Check sheet for the drawn part. Datum: minimum x, y, z corner. Units: mm. Give positions to 0.01 mm unless a question says otherwise; leave off trailing zeros. Write each loop counter-clockwise with the first axis right and the second up, starting at its lowest first coordinate (ties: lowest second). Pieces come first, ordered by that corner, then holes. Notation, with made-up numbers: (14, -14) - (43, -14) arc R17 cw to (43, 6) - close; hole circle Ø2 at (-28.75, 17). An arc over 180 degrees is marked (long way). Use a Markdown table: item, result.
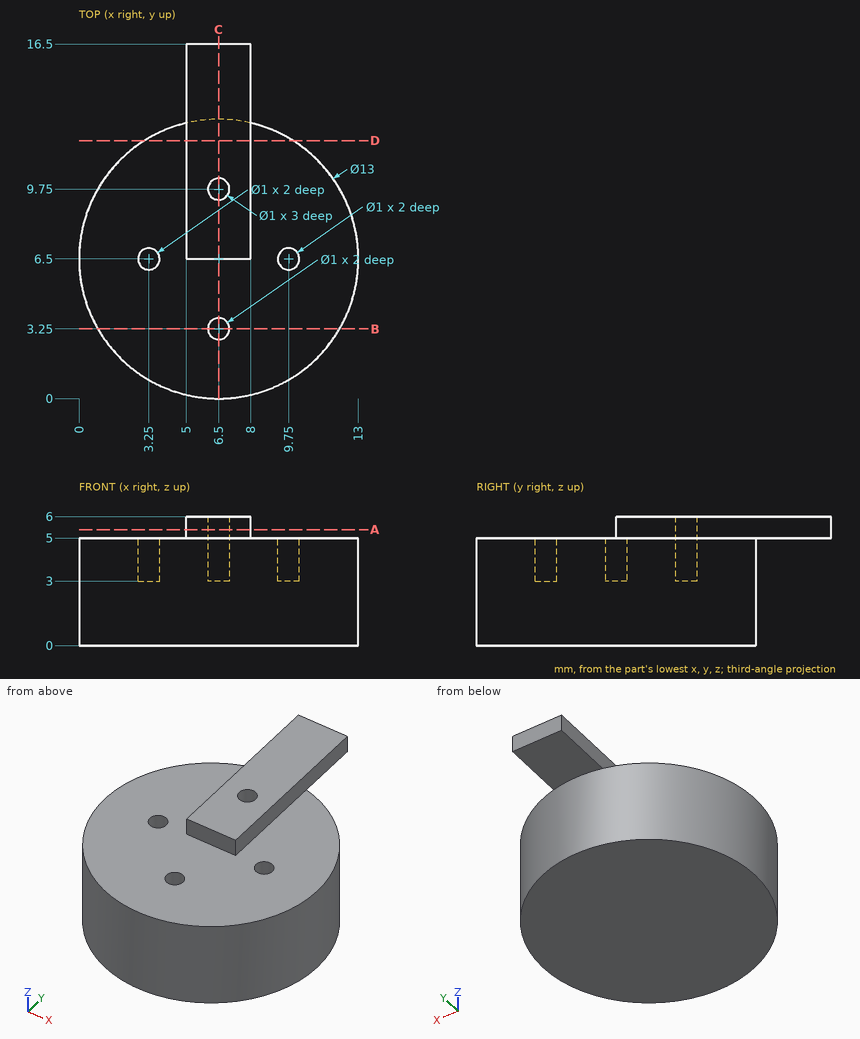
1) Material ranges on L1, parallel to X at y = 6.5, z = 3.55; L2, parallel to Z at x = 6.5, y = 15.25, recorded low to high. Write a range as from..to.
Working result:
| item | result |
|---|---|
| L1 | x = 0..2.75, 3.75..9.25, 10.25..13 |
| L2 | z = 5..6 |
2) Section check B-B on y = 3.25. Record the boundary of the cut face in (x, z), then the cut area to 3 significant figures.
Working result:
| item | result |
|---|---|
| outline | (0.87, 0) - (12.13, 0) - (12.13, 5) - (7, 5) - (7, 3) - (6, 3) - (6, 5) - (0.87, 5) - close |
| area | 54.3 mm² |
3) Section check D-D on y = 12. Record the boundary of the cut face in (x, z), then the cut area to 3 significant figures.
Working result:
| item | result |
|---|---|
| outline | (3.04, 0) - (9.96, 0) - (9.96, 5) - (8, 5) - (8, 6) - (5, 6) - (5, 5) - (3.04, 5) - close |
| area | 37.6 mm² |
4) Section check A-A on z = 5.4. Record the boundary of the cut face in (x, y).
Working result:
| item | result |
|---|---|
| outline | (5, 6.5) - (8, 6.5) - (8, 16.5) - (5, 16.5) - close; hole circle Ø1 at (6.5, 9.75) |
5) Depth check by flat-ended pin: P1, Ø2, axis at x = 1.5, z = 4, coming from the -Y side; P2, Ø0.8, axis at x = 6.5, y = 3, coming from the +Z side; P3, Ø1.1, axis at x = 7, z = 5.5, coming from the -Y side. Enter the tip coordinate at first touch or a pass-through.
Working result:
| item | result |
|---|---|
| P1 | stops at y = 1.38 |
| P2 | stops at z = 5 |
| P3 | stops at y = 0.01 |
6) Section check C-C on x = 6.5. Record the boundary of the cut face in (y, z), then the cut area to 3 significant figures.
Working result:
| item | result |
|---|---|
| outline | (0, 0) - (13, 0) - (13, 5) - (16.5, 5) - (16.5, 6) - (10.25, 6) - (10.25, 3) - (9.25, 3) - (9.25, 6) - (6.5, 6) - (6.5, 5) - (3.75, 5) - (3.75, 3) - (2.75, 3) - (2.75, 5) - (0, 5) - close |
| area | 70.0 mm² |
